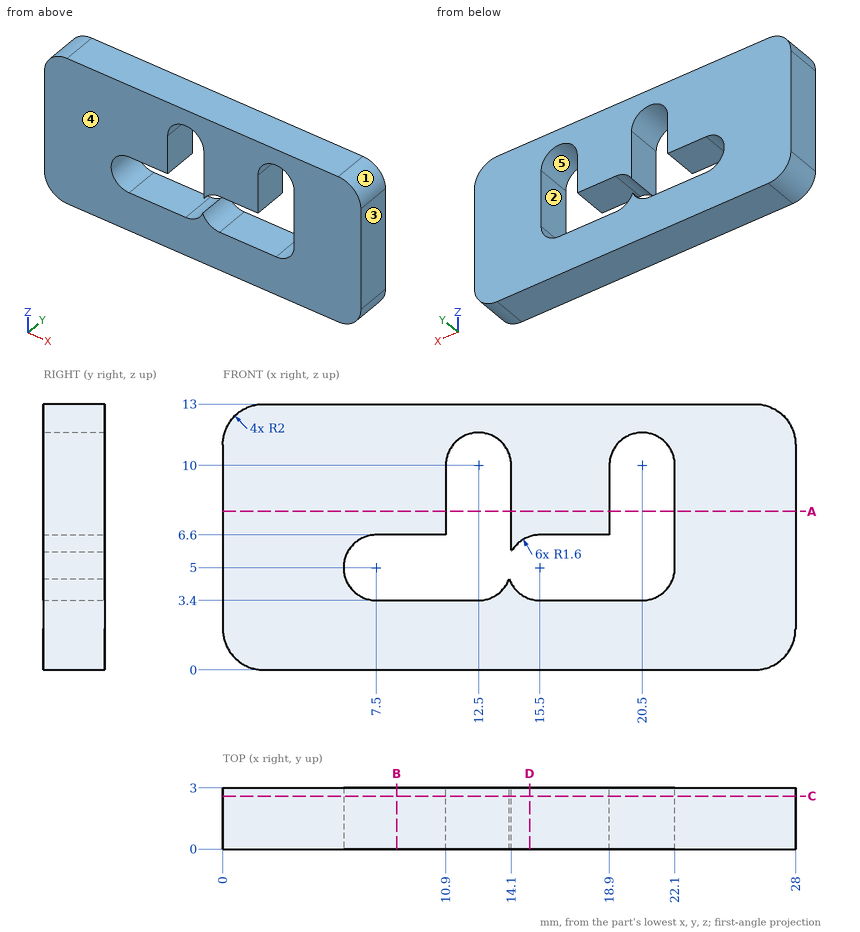
The drawing under review shows one solid part. Ordinate dimensions are in mm from its lowest x, y, z. A direction names the side the tool comes from. Round coordinates to 2 decimals unless told otherwise and drop trailing zeros. Write each loop counter-clockwise with the first axis right and the second up, starting at its lowest first coordinate (ties: lowest second). Pieces come first, ordered by that corner, then holes.
(1) We need section C-C on y = 2.6. Give the boundary of the cut face in (x, z).
(2) We need section A-A on z = 7.75. Give the boundary of the cut face in (x, y).
(3) Machinability: for the marked faces 4 and 5, which of the approach directions +Z, -Z, +X, -X, +Y, -Y give a long, thin tool a straight path to every point of the face, cutting with its end or side? Answer none if there is none.
(4) Mouldability with a two-part tool opening along Z and no side actions: class the marked faces 1, 2 and 3 as +Z half, -Z half, draft (parallel to the pull), parting line (faces both ways), or undercut.
(5) We need section B-B on x = 8.5. Give the boundary of the cut face in (y, z).
(6) We need section D-D on x = 15. Give the boundary of the cut face in (y, z), and give its area (3 significant figures).
(7) Wall thickness on L1, parallel to X at y = 2.3, z = 7.25; L2, parallel to Z at x = 15.5, y = 1.75; L3, parallel to Z at x = 11.25, y = 1.6: over which ranges is each line inside the solid? List them lowest first.
Findings below:
1. outline: (0, 2) arc R2 ccw to (2, 0) - (26, 0) arc R2 ccw to (28, 2) - (28, 11) arc R2 ccw to (26, 13) - (2, 13) arc R2 ccw to (0, 11) - close; hole (7.5, 3.4) - (12.5, 3.4) arc R1.6 ccw to (14, 4.44) arc R1.6 ccw to (15.5, 3.4) - (20.5, 3.4) arc R1.6 ccw to (22.1, 5) - (22.1, 10) arc R1.6 ccw to (18.9, 10) - (18.9, 6.6) - (15.5, 6.6) arc R1.6 ccw to (14.1, 5.77) - (14.1, 10) arc R1.6 ccw to (10.9, 10) - (10.9, 6.6) - (7.5, 6.6) arc R1.6 ccw to start
2. outline: (0, 0) - (10.9, 0) - (10.9, 3) - (0, 3) - close; (14.1, 0) - (18.9, 0) - (18.9, 3) - (14.1, 3) - close; (22.1, 0) - (28, 0) - (28, 3) - (22.1, 3) - close
3. face 4: +Z, -Z, +X, -X, -Y
3. face 5: +Y, -Y
4. face 1: +Z half
4. face 2: undercut
4. face 3: draft
5. outline: (0, 0) - (3, 0) - (3, 3.4) - (0, 3.4) - close; (0, 6.6) - (3, 6.6) - (3, 13) - (0, 13) - close
6. outline: (0, 0) - (3, 0) - (3, 3.48) - (0, 3.48) - close; (0, 6.52) - (3, 6.52) - (3, 13) - (0, 13) - close
6. area: 29.9 mm2
7. L1: x = 0 to 10.9, 14.1 to 18.9, 22.1 to 28
7. L2: z = 0 to 3.4, 6.6 to 13
7. L3: z = 0 to 3.4, 11 to 13
